The listing builds one solid part. Answer for the finished solid, in the listing's coordinates (mm). A direction names the side the tool comes from. Give positions to 0.01 mm unless a question says otherwise; leave off trailing zeros. Order: outer loops, then holes, each group sorted by start corner. A loop starts at its lowest first (then second) coordinate and runs counter-clockwise, first axis right, second up. Notation, with made-up numbers: (89.5, -28.5) - (145.5, -28.5) arc R35 ccw to (145.5, 4.5) - close; hole circle Ø5 at (15, -13.5). An arc over 180 degrees is marked (long way). Use CSV: the item, a comma, the result in double quotes.
```python
from build123d import *

# Parameters (mm, degrees)
BOSS_EXTRUDE1_DEPTH  = 3.175
CUT_EXTRUDE1_DEPTH   = 4.175
FILLET1_R            = 1.27
FILLET1_OF_MIRROR1_R = 1.27


with BuildPart() as part:
    # Sketch1 → Boss-Extrude1 (new body)
    with BuildSketch(Plane(origin=(0, -9.743731804, 0), x_dir=(1, 0, 0), z_dir=(0, 1, 0))):
        Polygon((28.575, 57.450862399), (28.575, 28.875862399), (31.75, 28.875862399), (31.75, 0.300862399), (28.575, 0.300862399), (28.575, -28.274137601), (31.75, -28.274137601), (31.75, -56.849137601), (-31.75, -56.849137601), (-31.75, -28.274137601), (-28.575, -28.274137601), (-28.575, 0.300862399), (-31.75, 0.300862399), (-31.75, 28.875862399), (-28.575, 28.875862399), (-28.575, 57.450862399), (-31.75, 57.450862399), (-31.75, 71.738362399), (31.75, 71.738362399), (31.75, 57.450862399), align=None)
    extrude(amount=BOSS_EXTRUDE1_DEPTH)

    # Sketch2 → Cut-Extrude1 (cut, through all)
    with BuildSketch(Plane(origin=(0, -6.568731804, 0), x_dir=(1, 0, 0), z_dir=(0, 1, 0))):
        Polygon((-22.225, -50.499137601), (-6.35, -50.499137601), (-6.35, -34.624137601), align=None)
        Polygon((-22.225, -41.51888148), (-6.35, -25.64388148), (-22.225, -25.64388148), align=None)
        Polygon((-6.35, -3.41888148), (-22.225, -19.29388148), (-6.35, -19.29388148), align=None)
        Polygon((-22.225, 5.561374641), (-22.225, -10.313625359), (-6.35, 5.561374641), align=None)
        Polygon((-6.35, 27.786374641), (-22.225, 11.911374641), (-6.35, 11.911374641), align=None)
        Polygon((-22.225, 36.766630762), (-22.225, 20.891630762), (-6.35, 36.766630762), align=None)
        Polygon((-6.35, 58.991630762), (-22.225, 43.116630762), (-6.35, 43.116630762), align=None)
        Polygon((-22.225, 67.971886883), (-22.225, 52.096886883), (-6.35, 67.971886883), align=None)
    cut_extrude1 = extrude(amount=-CUT_EXTRUDE1_DEPTH, mode=Mode.SUBTRACT)

    # Fillet1
    fillet1_edges = [part.edges().sort_by_distance(p)[0] for p in [
        (-22.225, -8.156231804, 41.51888148),
        (-22.225, -8.156231804, 25.64388148),
        (-6.35, -8.156231804, 25.64388148),
        (-6.35, -8.156231804, -67.971886883),
        (-22.225, -8.156231804, -52.096886883),
        (-22.225, -8.156231804, -67.971886883),
        (-6.35, -8.156231804, -43.116630762),
        (-22.225, -8.156231804, -43.116630762),
        (-6.35, -8.156231804, -58.991630762),
        (-6.35, -8.156231804, -36.766630762),
        (-22.225, -8.156231804, -20.891630762),
        (-22.225, -8.156231804, -36.766630762),
        (-22.225, -8.156231804, 50.499137601),
        (-6.35, -8.156231804, 34.624137601),
        (-6.35, -8.156231804, 50.499137601),
        (-6.35, -8.156231804, -11.911374641),
        (-22.225, -8.156231804, -11.911374641),
        (-6.35, -8.156231804, -27.786374641),
        (-6.35, -8.156231804, -5.561374641),
        (-22.225, -8.156231804, 10.313625359),
        (-22.225, -8.156231804, -5.561374641),
        (-6.35, -8.156231804, 19.29388148),
        (-22.225, -8.156231804, 19.29388148),
        (-6.35, -8.156231804, 3.41888148),
    ]]
    fillet(fillet1_edges, radius=FILLET1_R)

    # Mirror1: Cut-Extrude1 across plane
    add(cut_extrude1.mirror(Plane(origin=(0, 0, 0), x_dir=(0, 0, 1), z_dir=(1, 0, 0))), mode=Mode.SUBTRACT)

    # Fillet1 of Mirror1
    fillet1_of_mirror1_edges = [part.edges().sort_by_distance(p)[0] for p in [
        (22.225, -8.156231804, 41.51888148),
        (22.225, -8.156231804, 25.64388148),
        (6.35, -8.156231804, 25.64388148),
        (6.35, -8.156231804, -67.971886883),
        (22.225, -8.156231804, -52.096886883),
        (22.225, -8.156231804, -67.971886883),
        (6.35, -8.156231804, -43.116630762),
        (22.225, -8.156231804, -43.116630762),
        (6.35, -8.156231804, -58.991630762),
        (6.35, -8.156231804, -36.766630762),
        (22.225, -8.156231804, -20.891630762),
        (22.225, -8.156231804, -36.766630762),
        (22.225, -8.156231804, 50.499137601),
        (6.35, -8.156231804, 34.624137601),
        (6.35, -8.156231804, 50.499137601),
        (6.35, -8.156231804, -11.911374641),
        (22.225, -8.156231804, -11.911374641),
        (6.35, -8.156231804, -27.786374641),
        (6.35, -8.156231804, -5.561374641),
        (22.225, -8.156231804, 10.313625359),
        (22.225, -8.156231804, -5.561374641),
        (6.35, -8.156231804, 19.29388148),
        (22.225, -8.156231804, 19.29388148),
        (6.35, -8.156231804, 3.41888148),
    ]]
    fillet(fillet1_of_mirror1_edges, radius=FILLET1_OF_MIRROR1_R)


solid = part.part
```
Item 1: The mould has two halves that part along Z. Classify faces 5 (the face through (-31.75, -8, -14)), 6 (the face through (-20.34, -8.18, -43.92)): +Z half, -Z half, draft (parallel to the pull), parting line (faces both ways), or undercut.
Taken from the geometry:
face 5,"draft"
face 6,"undercut"
Item 2: Find the intervals of material crossed by line 1 along X through (y, z) = (-7.15, -13); line 2 along X through (y, z) = (-7, 34) (3 decimals); line 3 along X through (y, z) = (-9.05, -23.5), in increasing order.
Taken from the geometry:
line 1,"-31.75 to -20.42, -6.36 to 6.36, 20.42 to 31.75"
line 2,"-31.75 to -22.225, -14.706 to 14.706, 22.225 to 31.75"
line 3,"-31.75 to -22.14, -19.62 to -10.64, -6.35 to 6.35, 10.64 to 19.62, 22.14 to 31.75"
Item 3: Each of these flat-tipped pins is pushed along its axis until it touches: pin 1 (6 mm diameter, centred on x = 16, z = 14.5, fed in from +Y); pin 2 (1 mm diameter, centred on y = -8, z = 9.5, fed in from -X) (3 decimals); pin 3 (1.6 mm diameter, centred on y = -9, z = -48.5, fed in from +X) (3 decimals). Where does it stop, or does it pass through?
Taken from the geometry:
pin 1,"y = -6.57"
pin 2,"x = -28.575"
pin 3,"x = 28.575"
Item 4: The part is cut by section A-A (z = -16). Give the vertices of the cut face in (x, y).
Taken from the geometry:
outline,"(-31.75, -9.74) - (-18.14, -9.74) - (-18.14, -6.57) - (-31.75, -6.57) - close; (-6.35, -9.74) - (6.35, -9.74) - (6.35, -6.57) - (-6.35, -6.57) - close; (18.14, -9.74) - (31.75, -9.74) - (31.75, -6.57) - (18.14, -6.57) - close"
Item 5: The part is cut by section B-B (y = -9). Count the separate pieces of the cut face and the enclosed holes in it, and give its area (3 significant figures).
Taken from the geometry:
separate pieces,"1"
enclosed holes,"16"
area,"5,860 mm^2"
Item 6: The part is cut by section C-C (z = -52.5). Give the vertices of the cut face in (x, y) (3 decimals).
Taken from the geometry:
outline,"(-28.575, -9.744) - (-12.842, -9.744) - (-12.842, -6.569) - (-28.575, -6.569) - close; (-6.35, -9.744) - (6.35, -9.744) - (6.35, -6.569) - (-6.35, -6.569) - close; (12.842, -9.744) - (28.575, -9.744) - (28.575, -6.569) - (12.842, -6.569) - close"
Item 7: Which of the six approach directions +Z, -Z, +X, -X, +Y, -Y give full straight-line access (tool end or side, diameter ignored) to faces 1 (the face through (-30, -8, -0.301)), 2 (the face through (30, -8, 28.274)), 3 (the face through (-31.75, -8, 43)), 4 (the face through (-8.251, -8.178, -4.797))?
Taken from the geometry:
face 1,"-X, +Y, -Y"
face 2,"+X, +Y, -Y"
face 3,"+Z, -Z, -X, +Y, -Y"
face 4,"+Y, -Y"
